Design review of the part built by this model. Coordinates are the model's own, in mm. Round coordinates to 2 decimals unless told otherwise and drop trailing zeros. Loops run counter-clockwise (first coordinate to the right, second up) from the corner with the lowest first, then second, coordinate; pieces in that order, holes last. Notation, with made-up numbers: (26.5, 30) - (32.5, 30) arc R19 cw to (32.5, 65) - close; hole circle Ø10 at (3, -19.75). An arc over 180 degrees is marked (long way). Answer as CSV lines item,"result". Start each with the question number.
(1) For P1, Ø1.5, axis at x = 1.5, z = -55, coming from the +Y side; P2, Ø6.5, axis at y = 66.5, z = 0, coming from the +X side; P3, Ø3, axis at x = 4, y = 57.5, coming from the +Z side; P4, Ø1, axis at x = 2.5, y = -28.5, coming from the -Z side, all flat-tipped, find the tip position at first contact; note any pin that passes through.
(2) Consider section A-A (z = 0). Give the boundary of the cut face in (x, y), and give its area (4 significant figures).
(3) Wall thickness on L1, parallel to Z at x = 2.05, y = 0; L2, parallel to Z at x = 1.75, y = -33.25; L3, parallel to Z at x = 4.55, y = 13: over which ranges is each line inside the solid? List them lowest first.
(4) Consider section D-D (x = 2.6). Give the boundary of the cut face in (y, z).
(5) Consider section C-C (z = -16.5). Give the boundary of the cut face in (x, y).
(6) Consider section B-B (y = 0). Give the boundary of the cut face in (x, z), and give its area (4 significant figures).
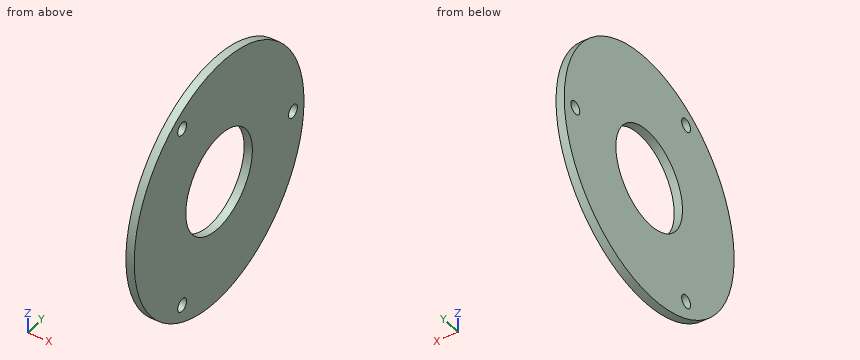
Autodesk Inventor part; units mm, degrees
ref_plane "YZ Plane" through (0, 0, 0) normal (1, 0, 0) x (0, 1, 0)
ref_plane "XZ Plane" through (0, 0, 0) normal (0, 1, 0) x (-1, 0, 0)
ref_plane "XY Plane" through (0, 0, 0) normal (0, 0, 1) x (1, 0, 0)
sketch "Sketch1" plane through (0, 0, 0) normal (1, 0, 0) x (0, 1, 0)
  circle A0 centre (0, 0) radius 30
  circle A1 centre (0, 0) radius 76.45
  dimension "d11" = 152.9
  dimension "d12" = 60
extrude "Extrusion1" add sketch "Sketch1" along normal blind 5
sketch "Sketch3" plane through (5, 0, 0) normal (1, 0, 0) x (0, 0, -1)
  circle A0 centre (0, 0) radius 66.5
  circle A1 centre (0, 66.5) radius 4
  circle A2 centre (-57.5907, -33.25) radius 4
  circle A3 centre (57.5907, -33.25) radius 4
  dimension "d23" = 133
  dimension "d24" = 8
  dimension "d45" = 360
extrude "Extrusion4" cut sketch "Sketch3" against normal through all contours A1 A0 | A0 A1 | A3 A0 | A0 A3 | A2 A0 | A0 A2
thread "Thread1"
thread "Thread5"
thread "Thread6"
properties part number "AsfaleiaDIpteroy"
Determined:
1,P1,"stops at y = 53.87"
1,P2,"passes through"
1,P3,"stops at z = 52.04"
1,P4,"stops at z = -71.14"
2,outline,"(0, -76.45) - (5, -76.45) - (5, -30) - (0, -30) - close; (0, 30) - (5, 30) - (5, 62.5) - (0, 62.5) - close; (0, 70.5) - (5, 70.5) - (5, 76.45) - (0, 76.45) - close"
2,area,"424.5 mm^2"
3,L1,"z = -76.45 to -30, 30 to 76.45"
3,L2,"z = -68.84 to -61.59, -53.59 to 53.59, 61.59 to 68.84"
3,L3,"z = -75.34 to -27.04, 27.04 to 75.34"
4,outline,"circle Ø152.9 at (0, 0); hole circle Ø8 at (-33.25, -57.59); hole circle Ø8 at (-33.25, 57.59); hole circle Ø60 at (0, 0); hole circle Ø8 at (66.5, 0)"
5,outline,"(0, -74.65) - (5, -74.65) - (5, -25.05) - (0, -25.05) - close; (0, 25.05) - (5, 25.05) - (5, 74.65) - (0, 74.65) - close"
6,outline,"(0, -76.45) - (5, -76.45) - (5, -30) - (0, -30) - close; (0, 30) - (5, 30) - (5, 76.45) - (0, 76.45) - close"
6,area,"464.5 mm^2"
